For this review, take the finished solid that the model builds, in its own axes (mm). A direction names the side the tool comes from. Give positions to 0.01 mm unless a question says otherwise; leave off trailing zeros. Write each loop counter-clockwise with the first axis right and the second up, starting at its lowest first coordinate (ties: lowest second). Pieces come first, ordered by that corner, then holes. Notation, with made-up numbers: M -31.5,53.25 L -13.5,53.25 A9 cw -13.5,57.25 Z; hole C 53.5,8 d5. An arc over 180 degrees is marked long. Write item = value, one per line.
Autodesk Inventor part; units mm, degrees
ref_plane "Work Plane1" through (30.1625, 0, 0) normal (0, 0, -1) x (1, 0, 0)
ref_plane "YZ Plane" through (0, 0, 0) normal (1, 0, 0) x (0, 1, 0)
ref_plane "XZ Plane" through (0, 0, 0) normal (0, 1, 0) x (-1, 0, 0)
sketch "Sketch1" plane through (0, 0, 0) normal (0, 0, 1) x (1, 0, 0)
  line L0 (-3, 0) -> (6, 0)
  line L1 (6, 0) -> (6, 2.5)
  line L2 (6, 2.5) -> (1.6, 2.5)
  line L3 (1.6, 2.5) -> (1.1091, 2.0095)
  line L4 (1.1091, 2.0095) -> (0, 2.0095)
  line L5 (0, 2.0095) -> (0, 5)
  line L6 (-4.8, 0) -> (7.8, 0)
  line L7 (0, -1) -> (0, 6)
  line L8 (-3, 0) -> (-3, 4.9995)
  line L9 (0, 5) -> (-3, 4.9995)
  line L10 (1.6, 2.5) -> (0, 2.5) construction
  dimension "d0" = 6
  dimension "d1" = 4.4
  dimension "d2" = 0.4909
  dimension "d3" = 3
  dimension "d4" = 5
  dimension "d5" = 4.019
  dimension "d9" = 10
  dimension "d10" = 0.01
revolve "Body" add sketch "Sketch1" angle 360 about axis through (-3, 0, 0) along (1, 0, 0)
sketch "Sketch2" plane through (-3, 0, 0) normal (-1, 0, 0) x (0, 0, 1)
  circle A0 centre (0, 0) radius 5
  line L0 (0, 0) -> (0, 4.9995)
  line L1 (-5, 0.755) -> (5, 0.755)
  line L2 (5, 0.755) -> (5, -0.755)
  line L3 (5, -0.755) -> (-5, -0.755)
  line L4 (-5, -0.755) -> (-5, 0.755)
  line L5 (-5, 0) -> (5, 0) construction
  line L6 (0, 0.755) -> (0, -0.755) construction
  dimension "d11" = 1.51
  dimension "d12" = 10
fillet "Fillet1" radius 2 1 edges at (-3, -4.9995, 0)
extrude "Slot" cut sketch "Sketch2" against normal blind 1.2 contours A0 L3 L1 | L2 L3 A0 | A0 L1 L2 | L3 L4 A0 | A0 L4 L1
thread "Thread"
chamfer "Chamfer1" distance 0.4908 distance2 0.4909 1 edges at (6, -2.5, 0) measured on face at (6, -0.1451, 0.646)
ref_plane "Work Plane1" through (30.1625, 0, 0) normal (0, 0, -1) x (1, 0, 0)
equation "\"d11\" = SBR"
equation "\"d12\" = KOD"
equation "\"d14\" = RR"
equation "\"d19\" = STI"
equation "\"d15\" = GEL"
equation "\"d17\" = -0.5 * SPD + 0.5 * GD"
equation "\"d0\" = NLG"
equation "\"d1\" = GEL"
equation "\"d3\" = KOH"
equation "\"d4\" = GD"
equation "\"d5\" = BDM"
equation "\"d9\" = KOD"
equation "\"d10\" = KEWI"
equation "\"GD\" = NND"
equation "\"NLG\" = 6"
equation "\"GEL\" = 4.4"
equation "\"KOD\" = 10"
equation "\"KOH\" = 3"
equation "\"GAL\" = 0.61345 * PTC"
equation "\"SPD\" = NND - 1.2269 * PTC"
equation "\"BDM\" = 4.019"
equation "\"GUL\" = 0.61345 * PTC"
equation "\"RR\" = 2"
equation "\"SBR\" = 1.51"
equation "\"STI\" = 1.2"
equation "\"KEWI\" = 0.01deg"
equation "\"PTC\" = 0.8"
equation "\"THREADDIA\" = 5"
equation "\"TOA\" = 30deg"
equation "\"NND\" = 5"
equation "\"RR1\" = 0.35"
equation "\"GD1\" = THREADDIA - 1.2269 * PTC"
properties part number "AS 1427 - M5 x 6" material "Steel, Mild"
1. The part is to be moulded in two halves that separate along Y. For faces 5 (the face through (0.547, 1.917, -0.604)), 6 (the face through (-3, 2, 0)), 7 (the face through (-2, -0.755, 0)), say which applies: +Y half, -Y half, draft (parallel to the pull), parting line (faces both ways), or undercut.
Responses:
face_5 = parting line
face_6 = draft
face_7 = undercut
2. We need section A-A, the plane y = 0. Write out the cut boundary in (x, z).
Responses:
outline = M -1.8,-4.83 A2 ccw -1,-5 L 0,-5 L 0,-2.01 L 1.11,-2.01 L 1.6,-2.5 L 5.51,-2.5 L 6,-2.01 L 6,2.01 L 5.51,2.5 L 1.6,2.5 L 1.11,2.01 L 0,2.01 L 0,5 L -1,5 A2 ccw -1.8,4.83 Z
3. Insertion check: P1, Ø0.6, axis at x = -2.5, z = 0.5, coming from the -Y side; P2, Ø0.5, axis at y = 0, z = 1.5, coming from the -X side; P3, Ø5, axis at x = -2, z = -3, coming from the -Y side. Each pin has a flat end and moves straight along its axis. Give the tip position at first contact, or say it passes through.
Responses:
P1 = -4.57
P2 = -1.8
P3 = -4.95
4. We need section C-C, the plane x = -2.5. Write out the cut boundary in (y, z) (3 decimals).
Responses:
outline = M -0.755,-4.256 L -0.755,4.256 A4.323 ccw Z; M 0.755,-4.256 A4.323 ccw 0.755,4.256 Z
5. We need section B-B, the plane z = 0. Write out the cut boundary in (x, y) (1 decimal).
Responses:
outline = M -3,-3 A2 ccw -1,-5 L 0,-5 L 0,-2 L 1.1,-2 L 1.6,-2.5 L 5.5,-2.5 L 6,-2 L 6,2 L 5.5,2.5 L 1.6,2.5 L 1.1,2 L 0,2 L 0,5 L -1,5 A2 ccw -3,3 L -3,0.8 L -1.8,0.8 L -1.8,-0.8 L -3,-0.8 Z
6. Machinability: for faces 1 (the face through (6, 0, 0)), 2 (the face through (-1.8, 0, 0)), 3 (the face through (3.53, -0.54, 2.44)), 4 (the face through (0, 2.2, 0.1)), which of the approach directions +Z, -Z, +X, -X, +Y, -Y give a long, thin tool a straight path to every point of the face, cutting with its end or side? Answer none if there is none.
Responses:
face_1 = +Z, -Z, +X, +Y, -Y
face_2 = +Z, -Z, -X
face_3 = +X
face_4 = none
7. For line 1 along X through (y, z) = (-1.75, 2.5); line 2 along Y through (x, z) = (-2.25, 1) (3 decimals); line 3 along X through (y, z) = (-0.5, -3.75), list the stretches that pass through material, from the lowest coordinate up. Write a range as from..to.
Responses:
line_1 = -3..0
line_2 = -4.45..-0.755, 0.755..4.45
line_3 = -1.8..0
8. We need section D-D, the plane x = 4.75. Write out the cut boundary in (y, z), then the cut area to 3 significant figures.
Responses:
outline = C 0,0 d5
area = 19.6 mm2
